Autodesk Inventor part; units mm, degrees
ref_plane "IDS_WORKPLANE{1}" through (-7.5, 0, 0) normal (1, 0, 0) x (0, 0, -1)
ref_plane "Work Plane2" through (69.85, 0, 0) normal (0, 0, -1) x (1, 0, 0)
ref_plane "YZ Plane" through (0, 0, 0) normal (1, 0, 0) x (0, 1, 0)
sketch "Skizze1" plane through (0, 0, 0) normal (0, 0, 1) x (1, 0, 0)
  line L0 (-2.57, 0) -> (13, 0)
  line L1 (13, 0) -> (13, 5)
  line L2 (13, 5) -> (0, 5)
  line L3 (0, 5) -> (0, 10)
  line L4 (-12.0526, 0) -> (17.1754, 0)
  line L5 (0, -2.0361) -> (0, 12.2164)
  line L6 (-7.5, 3.4435) -> (-5.0836, 3.4435) construction
  line L7 (-7.5, 0) -> (-2.57, 0)
  line L8 (0, 0) -> (-2.57, 0)
  line L9 (-7.5, 0) -> (-7.5, 10)
  arc A0 (-4.3649, 10) -> (-7.5, 3.4435) centre (8.1251, 0) ccw
  line L10 (-7.5, 10) -> (0, 10)
  dimension "d0" = 13
  dimension "d1" = 10
  dimension "d2" = 20
  dimension "d4" = 6.887
  dimension "d13" = 7.5
  dimension "d14" = 4.93
  dimension "d46" = 16
  dimension "d47" = 0
revolve "Körper" add sketch "Skizze1" angle 360 about axis through (-2.57, 0, 0) along (1, 0, 0) contours L4 L9 A0 L10 L3 L5 L0 | L5 L2 L1 L0
ref_plane "IDS_WORKPLANE{1}" through (-7.5, 0, 0) normal (1, 0, 0) x (0, 0, -1)
sketch "Skizze2" plane through (-7.5, 0, 0) normal (1, 0, 0) x (0, 0, -1)
  line L0 (0, -14) -> (0, 14)
  line L1 (14, 0) -> (-14, 0)
  line L2 (-1.932, 1.932) -> (1.932, 1.932)
  line L3 (1.932, 1.932) -> (1.932, -1.932)
  line L4 (1.932, -1.932) -> (-1.932, -1.932)
  line L5 (-1.932, -1.932) -> (-1.932, 1.932)
  line L6 (0, 1.932) -> (0, -1.932) construction
  line L7 (-1.932, 0) -> (1.932, 0) construction
  dimension "d7" = 3.864
  dimension "d9" = 3.864
extrude "Extrusion" cut sketch "Skizze2" along normal blind 4.93
fillet "Rundung1" radius 1.932 4 edges at (-2.57, 0, -1.932) (-2.57, -1.932, 0) (-2.57, 0, 1.932) (-2.57, 1.932, 0)
chamfer "Fase1" distance 0.493 angle 45 4 edges at (-7.5, 1.932, 0) (-7.5, 0, -1.932) (-7.5, -1.932, 0) (-7.5, 0, 1.932)
thread "Gewinde"
chamfer "Fase2" distance 1.32 distance2 0.9202 1 edges at (13, -5, 0) measured on face at (13, -0.8193, -0.3214)
ref_plane "Work Plane2" through (69.85, 0, 0) normal (0, 0, -1) x (1, 0, 0)
fillet "Rundung2" radius 0.4 1 edges at (0, -5, 0)
equation "\"d7\" = KOM - 0.2 * STI"
equation "\"d9\" = KOM - 0.2 * STI"
equation "\"d0\" = NLG"
equation "\"d1\" = GD"
equation "\"d2\" = KOD"
equation "\"d4\" = 1.42 * KOM"
equation "\"d13\" = KOH"
equation "\"d14\" = STI"
equation "\"d46\" = KR"
equation "\"d48\" = STI"
equation "\"d50\" = -0.1 * STI + 0.5 * KOM"
equation "\"d51\" = 0.1 * STI"
equation "\"d18\" = GEL"
equation "\"d20\" = -0.5 * SPD + 0.5 * GD"
equation "\"d21\" = GUL"
equation "\"d44\" = R"
equation "\"GD\" = 10"
equation "\"NLG\" = 13"
equation "\"GEL\" = 11.5"
equation "\"KOD\" = 20"
equation "\"KOH\" = 7.5"
equation "\"SPD\" = 7.36"
equation "\"KR\" = 16"
equation "\"RR\" = 3.2"
equation "\"GUL\" = 0.61345 * PTC"
equation "\"KEWI\" = 0"
equation "\"SDM\" = 4.86"
equation "\"STI\" = 4.93"
equation "\"d6\" = -KOH"
equation "\"R\" = 0.4"
equation "\"KOM\" = 4.85"
equation "\"KOP\" = 16"
equation "\"PTC\" = 1.5"
properties part number "ANSI B18.6.7M - M10x1,5 x 13, SRPHMSTIM" material "Stahl, weich"
Source: CAD feature listing. Evaluate the final solid. Frame: model axes, mm. A direction names the side the tool comes from. Round coordinates to 2 decimals unless told otherwise and drop trailing zeros. Order: outer loops, then holes, each group sorted by start corner. A loop starts at its lowest first (then second) coordinate and runs counter-clockwise, first axis right, second up. Notation, with made-up numbers: (-19, -16) - (36, -16) arc R33 ccw to (36, 19) - close; hole circle Ø3 at (-27, 3.25). An arc over 180 degrees is marked (long way). Use a Markdown table: item, result. Add a question column.
1. First-contact query: pin 1 (2 mm diameter, centred on x = -6, z = -1, fed in from -Y); pin 2 (5 mm diameter, centred on x = 9.5, y = 4, fed in from +Z); pin 3 (4 mm diameter, centred on x = 9, y = 3, fed in from +Z). Flat tips, straight axial feed; report the tip coordinate or a pass-through.
2. Mould query, pull axis Z, two halves, no side actions, for faces 4 (the cylindrical face through (-3.411, -1.595, 0.027)), 5 (the flat face through (13, 0, 0)), 6 (the cylindrical face through (-2.15, -2.17, -9.76)). Classes: +Z half, -Z half, draft (parallel to the pull), parting line (faces both ways), or undercut.
3. Line query: probe 1 along Z at (x, y) = (-4, 1.5); probe 2 along X at (y, z) = (-1, -1.5); probe 3 along Z at (x, y) = (0.5, 0). Output: solid intervals per line, ascending.
4. Section query A-A (x = -1). Return the cut outline in (y, z).
5. Set-up query: faces 1 (the flat face through (-6, 0, -1.932)), 2 (the flat face through (-7.5, 0, -3)), 3 (the flat face through (0, 4, -4)). Return all of +Z, -Z, +X, -X, +Y, -Y with unobstructed straight access to the full face (end or side cutting, diameter ignored); none if empty.
6. Section query B-B (x = 4). Return the cut outline in (y, z), then the cut area to 3 significant figures.
Derived:
| question | item | result |
|---|---|---|
| 1 | pin 1 | y = -9.1 |
| 1 | pin 2 | z = 4.77 |
| 1 | pin 3 | z = 4.9 |
| 2 | face 4 | undercut |
| 2 | face 5 | draft |
| 2 | face 6 | parting line |
| 3 | probe 1 | -9.89 to -1.87, 1.87 to 9.89 |
| 3 | probe 2 | -3.28 to 13 |
| 3 | probe 3 | -5 to 5 |
| 4 | outline | circle Ø20 at (0, 0) |
| 5 | face 1 | -X |
| 5 | face 2 | +Z, -Z, -X, +Y, -Y |
| 5 | face 3 | +X |
| 6 | outline | circle Ø10 at (0, 0) |
| 6 | area | 78.5 mm2 |
